Autodesk Inventor part; units mm, degrees
ref_plane "YZ Plane" through (0, 0, 0) normal (1, 0, 0) x (0, 1, 0)
ref_plane "XZ Plane" through (0, 0, 0) normal (0, 1, 0) x (-1, 0, 0)
ref_plane "XY Plane" through (0, 0, 0) normal (0, 0, 1) x (1, 0, 0)
sketch "Sketch2" plane through (0, 0, 0) normal (0, 0, 1) x (1, 0, 0)
  line L0 (2.5, 0) -> (2.5, 5)
  line L1 (2.5, 5) -> (4, 5)
  line L2 (4, 5) -> (4, 45)
  line L3 (0, 0) -> (0, 45)
  line L4 (0, 0) -> (2.5, 0)
  line L5 (4, 45) -> (0, 45)
  point P0 (0, 25)
  dimension "d2" = 5
  dimension "d3" = 40
  dimension "d4" = 8
  dimension "d5" = 5
revolve "Revolution1" add sketch "Sketch2" angle 360 about axis through (0, 0, 0) along (0, 1, 0)
thread "Thread1"
chamfer "Chamfer1" distance 0.5 angle 45 2 edges at (-4, 45, 0) (-2.5, 0, 0)
properties part number "OringM5Wrench" material "Stainless Steel, 440C"
The model under review builds one solid part; all positions refer to its coordinate system, in mm. A direction names the side the tool comes from. Coordinates: 2 decimals unless noted, no trailing zeros. Write each loop counter-clockwise with the first axis right and the second up, starting at its lowest first coordinate (ties: lowest second). Pieces come first, ordered by that corner, then holes. Notation, with made-up numbers: (-21.75, 87.5) - (-0.75, 87.5) arc R30 ccw to (-0.75, 122.5) - close; hole circle Ø7 at (39, 43). An arc over 180 degrees is marked (long way). Answer as CSV lines item,"result".
(1) We need section B-B (x = 0). Give the boundary of the cut face in (y, z).
Data:
outline,"(0, -2) - (0.5, -2.5) - (5, -2.5) - (5, -4) - (44.5, -4) - (45, -3.5) - (45, 3.5) - (44.5, 4) - (5, 4) - (5, 2.5) - (0.5, 2.5) - (0, 2) - close"
(2) Clearance check with a flat-ended pin moving along its axis: pin 1 Ø2 at (x, z) = (3, 0.5) entering from -Y. State where the tip first meets the part, or that it passes through.
Data:
pin 1,"stops at y = 0.04"
(3) For line 1 along Y through (x, z) = (-2, -2.5); line 2 along Z through (x, y) = (0.25, 40.5); line 3 along Z through (x, y) = (1, 37), list the stretches that pass through material, from the lowest coordinate up. Write a range as [from, to].
Data:
line 1,"y = [5, 45]"
line 2,"z = [-3.99, 3.99]"
line 3,"z = [-3.87, 3.87]"
(4) Tool access review of faces 1 (the flat face through (0, 0, 0)), 2 (the cylindrical face through (-0.54, 2.78, 2.44)): name each direction out of +Z, -Z, +X, -X, +Y, -Y from which nothing blocks a thin tool from reaching the whole face with its end or side.
Data:
face 1,"+Z, -Z, +X, -X, -Y"
face 2,"-Y"
(5) We need section A-A (z = 0). Give the boundary of the cut face in (x, y).
Data:
outline,"(-4, 5) - (-2.5, 5) - (-2.5, 0.5) - (-2, 0) - (2, 0) - (2.5, 0.5) - (2.5, 5) - (4, 5) - (4, 44.5) - (3.5, 45) - (-3.5, 45) - (-4, 44.5) - close"
(6) We need section C-C (y = 6.5). Give the boundary of the cut face in (x, z), plus the area to 3 significant figures.
Data:
outline,"circle Ø8 at (0, 0)"
area,"50.3 mm2"
